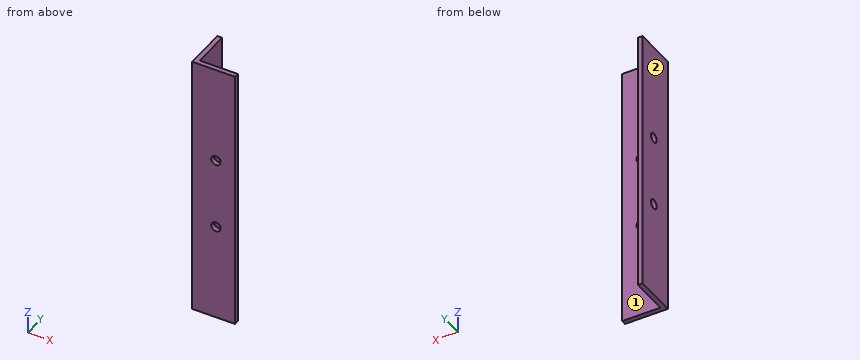
from build123d import *

# Parameters (mm, degrees)
F1_DEPTH = 56
F2_R     = 1
F3_DEPTH = 1
F4_R     = 1
F5_DEPTH = 1


with BuildPart() as f1:
    # F0 (on Top) → F1 (new body)
    with BuildSketch(Plane.XY):
        Polygon((0, 9), (0, 0), (9, 0), (9, 1), (1, 1), (1, 9), align=None)
    extrude(amount=F1_DEPTH)

    # F2 (on face) → F3 (cut, through all)
    with BuildSketch(Plane.XZ):
        with Locations((5, 35.5)):
            Circle(F2_R)
        with Locations((5, 20.5)):
            Circle(F2_R)
    extrude(amount=-F3_DEPTH, mode=Mode.SUBTRACT)

    # F4 (on face) → F5 (cut, through all)
    with BuildSketch(Plane(origin=(0, 0, 0), x_dir=(0, -1, 0), z_dir=(-1, 0, 0))):
        with Locations((-5, 35.5)):
            Circle(F4_R)
        with Locations((-5, 20.5)):
            Circle(F4_R)
    extrude(amount=-F5_DEPTH, mode=Mode.SUBTRACT)


solid = f1.part
Model file for the job. Use its own axes, mm. Face numbers are marked on the shaded views. A direction names the side the tool comes from. Give positions to 0.01 mm unless a question says otherwise; leave off trailing zeros. Loops run counter-clockwise (first coordinate to the right, second up) from the corner with the lowest first, then second, coordinate; pieces in that order, holes last. Notation, with made-up numbers: (81, -38.75) - (108, -38.75) arc R25 ccw to (108, -8.75) - close; hole circle Ø5 at (-40, -15). An arc over 180 degrees is marked (long way). Use one line per item in the form item = value.
(1) 3-axis set-ups, long thin cutter, end or side, ignore diameter. For the marked faces 1 and 2: which of +Z, -Z, +X, -X, +Y, -Y reach the whole face in a straight line?
Determined:
face_1 = +Z, -Z, +X, +Y
face_2 = +Z, -Z, -X, +Y, -Y
(2) Drill centre lines: L1, parallel to Z at x = 5, y = 0.65; L2, parallel to Y at x = 7.25, z = 14.5. Where is each one in solid material? Low to high.
Determined:
L1 = 0 to 19.5, 21.5 to 34.5, 36.5 to 56
L2 = 0 to 1
(3) Cut at A-A (y = 5). Give the cut face in (x, z).
Determined:
outline = (0, 0) - (1, 0) - (1, 19.5) - (0, 19.5) - close; (0, 21.5) - (1, 21.5) - (1, 34.5) - (0, 34.5) - close; (0, 36.5) - (1, 36.5) - (1, 56) - (0, 56) - close
(4) Cut at D-D (x = 8.5). Give the cut face in (y, z), then the cut area to 3 significant figures.
Determined:
outline = (0, 0) - (1, 0) - (1, 56) - (0, 56) - close
area = 56.0 mm^2
(5) Drop flat-ended pins along their axis: P1, Ø3, axis at x = 7, z = 34.5, coming from the +Y side; P2, Ø1.6, axis at x = 5, z = 20.5, coming from the +Y side; P3, Ø2, axis at y = 5.5, z = 10.5, coming from the +X side. Give the stop position or say it passes through.
Determined:
P1 = 1
P2 = through
P3 = 1
(6) Cut at B-B (z = 20.5). Give the cut face in (x, y), then the cut area to 3 significant figures.
Determined:
outline = (0, 0) - (4, 0) - (4, 1) - (1, 1) - (1, 4) - (0, 4) - close; (0, 6) - (1, 6) - (1, 9) - (0, 9) - close; (6, 0) - (9, 0) - (9, 1) - (6, 1) - close
area = 13.0 mm^2
